CAD build for the part. Positions are in the model's coordinates, mm. Face numbers are marked on the shaded views. A direction names the side the tool comes from. Coordinates: 2 decimals unless noted, no trailing zeros. Loops run counter-clockwise (first coordinate to the right, second up) from the corner with the lowest first, then second, coordinate; pieces in that order, holes last. Notation, with made-up numbers: (16, 27) -> (44, 27) arc R20 cw to (44, 43) -> close; hole circle Ø6 at (-15.5, -19.75). An arc over 180 degrees is marked (long way). Answer as a JSON object with one key per item and string values. Group by question number.
Autodesk Inventor part; units mm, degrees
ref_plane "YZ Plane" through (0, 0, 0) normal (1, 0, 0) x (0, 1, 0)
ref_plane "XZ Plane" through (0, 0, 0) normal (0, 1, 0) x (-1, 0, 0)
ref_plane "XY Plane" through (0, 0, 0) normal (0, 0, 1) x (1, 0, 0)
sketch "Sketch1" plane through (0, 0, 0) normal (0, 0, 1) x (1, 0, 0)
  line L0 (-21, 21) -> (21, 21)
  line L1 (21, 21) -> (21, -21)
  line L2 (21, -21) -> (-21, -21)
  line L3 (-21, -21) -> (-21, 21)
  line L4 (15.5, 15.5) -> (-15.5, 15.5) construction
  line L5 (-15.5, 15.5) -> (-15.5, -15.5)
  line L6 (-15.5, -15.5) -> (15.5, -15.5) construction
  line L7 (15.5, -15.5) -> (15.5, 15.5)
  circle A0 centre (-15.5, 15.5) radius 1.75
  circle A1 centre (15.5, 15.5) radius 1.75
  circle A2 centre (-15.5, -15.5) radius 1.75
  circle A3 centre (15.5, -15.5) radius 1.75
  point P0 (0, 0)
  point P1 (0, 0)
  dimension "d0" = 42
  dimension "d1" = 5.5
  dimension "d2" = 3.5
extrude "Extrusion1" add sketch "Sketch1" along normal blind 25
sketch "Sketch2" plane through (21, -21, 0) normal (1, 0, 0) x (0, 0, -1)
  line L0 (0, 42) -> (0, 0)
  line L1 (0, 42) -> (-25, 42)
  line L2 (-25, 0) -> (-25, 42)
  line L3 (0, 0) -> (-25, 0)
  point P0 (0, 21)
extrude "Extrusion2" add sketch "Sketch2" along normal blind 4.6
sketch "Sketch3" plane through (0, 0, 25) normal (0, 0, 1) x (1, 0, 0)
  circle A0 centre (15.5, 15.5) radius 1.75
  line L0 (25.6, 21) -> (25.6, -21)
  circle A1 centre (15.5, 15.5) radius 16.9
  line L1 (25.6, 15.5) -> (32.4, 15.5)
  point P0 (0, 0)
  dimension "d7" = 16.9
extrude "Extrusion3" add sketch "Sketch3" against normal up to surface (25 mm away)
sketch "Sketch4" plane through (-21, -21, 0) normal (0, -1, 0) x (1, 0, 0)
  line L0 (46.6, 0) -> (0, 0)
  circle A0 centre (32.1, 15) radius 3
  point P0 (21, 0)
  dimension "d11" = 11.1
  dimension "d12" = 15
  dimension "d13" = 6
extrude "Extrusion4" cut sketch "Sketch4" against normal blind 10
properties part number "TITAN MOCKUP"
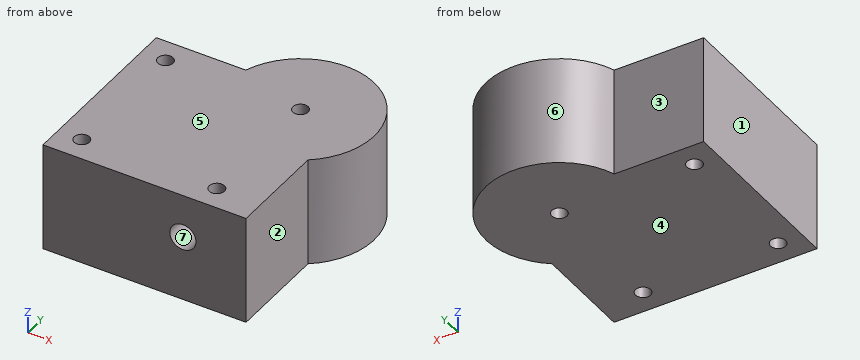
Item 1: 3-axis set-ups, long thin cutter, end or side, ignore diameter. For the marked faces 1, 2 and 3: which of +Z, -Z, +X, -X, +Y, -Y reach the whole face in a straight line?
Item 2: Band-saw the part on A-A, the plane x = 15.5. List the corners of the cut face in (y, z), and give its area (3 significant figures).
Item 3: Drill centre lines: L1, parallel to Y at x = 15.5, z = 16.75; L2, parallel to X at y = -15.5, z = 11.25. Where is each one in solid material? Low to high.
Item 4: Band-saw the part on C-C, the plane z = 4.5. List the corners of the cut face in (x, y).
Item 5: Band-saw the part on D-D, the plane z = 14.25. List the corners of the cut face in (x, y).
Item 6: Pull direction Z, two halves, no side cores. Call the marked faces 4, 5, 6 and 7: +Z half, -Z half, draft (parallel to the pull), parting line (faces both ways), or undercut.
Item 7: Flat gauge pins, fed straight in: P1, Ø5, axis at y = -8.5, z = 20, coming from the +X side; P2, Ø1.5, axis at x = 1, z = 11.5, coming from the +Y side; P3, Ø2, axis at x = -15.5, y = -15.5, coming from the +Z side; P4, Ø1.5, axis at x = 24.5, z = 8, coming from the +Y side. Where does each tip first touch, or does it go through?
Reply:
{
 "1": {"face 1": "+Z, -Z, -X, +Y, -Y", "face 2": "+Z, -Z, +X, -Y", "face 3": "+Z, -Z, -X, +Y"},
 "2": {"outline": "(-21, 0) -> (-17.25, 0) -> (-17.25, 25) -> (-21, 25) -> close; (-13.75, 0) -> (13.75, 0) -> (13.75, 25) -> (-13.75, 25) -> close; (17.25, 0) -> (32.4, 0) -> (32.4, 25) -> (17.25, 25) -> close", "area": "1,160 mm²"},
 "3": {"L1": "-21 to -17.25, -13.75 to 13.75, 17.25 to 32.4", "L2": "-21 to -17.25, -13.75 to 13.75, 17.25 to 25.6"},
 "4": {"outline": "(-21, -21) -> (25.6, -21) -> (25.6, 1.95) arc R16.9 ccw (long way) to (-0.48, 21) -> (-21, 21) -> close; hole circle Ø3.5 at (-15.5, -15.5); hole circle Ø3.5 at (-15.5, 15.5); hole circle Ø3.5 at (15.5, -15.5); hole circle Ø3.5 at (15.5, 15.5)"},
 "5": {"outline": "(-21, -21) -> (8.2, -21) -> (8.2, -11) -> (14, -11) -> (14, -14.59) arc R1.75 cw (long way) to (14, -16.41) -> (14, -21) -> (25.6, -21) -> (25.6, 1.95) arc R16.9 ccw (long way) to (-0.48, 21) -> (-21, 21) -> close; hole circle Ø3.5 at (-15.5, -15.5); hole circle Ø3.5 at (-15.5, 15.5); hole circle Ø3.5 at (15.5, 15.5)"},
 "6": {"face 4": "-Z half", "face 5": "+Z half", "face 6": "draft", "face 7": "undercut"},
 "7": {"P1": "x = 25.6", "P2": "y = 25.33", "P3": "through", "P4": "y = 30.25"}
}
